Geometry: final body of the model. Coordinates: model frame, mm. A direction names the side the tool comes from. Give positions to 0.01 mm unless a question says otherwise; leave off trailing zeros. Write each loop counter-clockwise with the first axis right and the second up, starting at its lowest first coordinate (ties: lowest second). Pieces come first, ordered by that corner, then holes.
Q1. Cut plane D-D on y = 79. Return the cut outline in (x, z).
Q2. Cut plane A-A on z = -107.95. Return the cut outline in (x, y), plus the area to 3 significant figures.
Q3. Draft query along Z for faces 1 (the face through (-117.96, -25.13, -26.78)), 2 (the face through (107.683, -49.491, 63.856)), 3 (the face through (-114.478, -49.491, -70.117)), 4 (the face through (-120, -91.44, -112)). Return one class per face: pulls with the +Z half, pulls with the -Z half, needs draft (parallel to the pull), parting line crosses it, or undercut.
Q4. Pin query (flat end, axial travel): pin 1 (4 mm diameter, centred on x = -62, z = 95, fed in from +Y); pin 2 (3 mm diameter, centred on y = -2, z = 18.5, fed in from -X); pin 3 (14.5 mm diameter, centred on x = 107.95, z = 107.95, fed in from +Y); pin 4 (10 mm diameter, centred on x = 98.5, z = -73.5, fed in from -Y). Return the tip coordinate at first contact, or that it passes through.
Q5. Cut plane B-B on x = 0. Return the cut outline in (y, z).
Q6. Reachability of faces 5 (the face through (114, -6.35, -7)), 6 (the face through (-1, -104.14, 82)), 7 (the face through (-108, -91.44, 117)) from +Z, -Z, +X, -X, +Y, -Y: full face, straight path, thin tool, end or side. Return the list, or none.
Q7. Cut plane C-C on z = 107.95. Return the cut outline in (x, y), plus the area to 3 significant figures.
Q8. Line query: L1, parallel to X at y = -15.5, z = -40.5; L2, parallel to Z at x = 111.76, y = -35; L3, parallel to Y at x = 39.5, z = -5.5. Output: solid intervals per line, ascending.
```python
from build123d import *

# Parameters (mm, degrees)
SKETCH1_R                = 101.6
SKETCH1_R_2              = 88.9
BOSS_EXTRUDE1_DEPTH      = 38.1
SKETCH2_W                = 254
SKETCH2_H                = 177.8
BOSS_EXTRUDE2_DEPTH      = 12.7
BOSS_EXTRUDE3_REACH      = 275.106
BOSS_EXTRUDE3_END_RADIUS = 101.6
SKETCH3_W                = 203.2
SKETCH3_H                = 38.1
SKETCH10_W               = 25.4
SKETCH10_H               = 88.9
BOSS_EXTRUDE5_DEPTH      = 97.79
SKETCH11_R               = 6.35
CUT_EXTRUDE1_DEPTH       = 38.1
RIB3_START               = -38.1
RIB3_DEPTH               = 38.1
BOSS_EXTRUDE6_DEPTH      = 25.4
BOSS_EXTRUDE7_DEPTH      = 25.4
SKETCH17_R               = 6.35
CUT_EXTRUDE2_DEPTH       = 25.4


# Read off the part's stored shape, not the designer's step: Rib3
with BuildPart() as part:
    # Sketch1 → Boss-Extrude1 (new body)
    with BuildSketch(Plane.XY):
        with Locations(Location((0, 0, 0), (0, 0, 180))):
            Circle(SKETCH1_R)
        with Locations(Location((0, 0, 0), (0, 0, 180))):
            Circle(SKETCH1_R_2, mode=Mode.SUBTRACT)
    extrude(amount=BOSS_EXTRUDE1_DEPTH)



with BuildPart() as body_2:
    # Sketch2 → Boss-Extrude2 (new body)
    with BuildSketch(Plane(origin=(0, -116.84, 0), x_dir=(1, 0, 0), z_dir=(0, 1, 0))):
        with Locations((0, -38.1)):
            Rectangle(SKETCH2_W, SKETCH2_H)
    extrude(amount=BOSS_EXTRUDE2_DEPTH)


with BuildPart() as part_1:
    add(part.part)

    add(body_2.part)  # Boss-Extrude3 merges body 2
    # Boss-Extrude3: up to this cylinder (the profile starts outside it)
    boss_extrude3_end = Plane(origin=(0, 0, 19.05), z_dir=(0, 0, -1)) * Cylinder(BOSS_EXTRUDE3_END_RADIUS, 754.412, mode=Mode.PRIVATE)
    # Sketch3 → Boss-Extrude3 (add, up to the surface)
    with BuildSketch(Plane(origin=(0, -104.14, 0), x_dir=(1, 0, 0), z_dir=(0, 1, 0)), mode=Mode.PRIVATE) as boss_extrude3_sk1:
        with Locations((0, -19.05)):
            Rectangle(SKETCH3_W, SKETCH3_H)
    boss_extrude3_tool1 = extrude(boss_extrude3_sk1.sketch, amount=BOSS_EXTRUDE3_REACH, mode=Mode.PRIVATE) - boss_extrude3_end
    add(boss_extrude3_tool1.solids().sort_by_distance((0, -104.14, 19.05))[0])

    # Sketch10 → Boss-Extrude5 (add)
    with BuildSketch(Plane(origin=(0, -104.14, 0), x_dir=(1, 0, 0), z_dir=(0, 1, 0))):
        with Locations((-114.3, 6.35)):
            Rectangle(SKETCH10_W, SKETCH10_H)
    boss_extrude5 = extrude(amount=BOSS_EXTRUDE5_DEPTH)

    # Mirror1: Boss-Extrude5 across plane
    add(boss_extrude5.mirror(Plane(origin=(0, 0, 0), x_dir=(0, 0, 1), z_dir=(1, 0, 0))))

    # Sketch11 → Cut-Extrude1 (cut)
    with BuildSketch(Plane(origin=(0, -6.35, 0), x_dir=(1, 0, 0), z_dir=(0, 1, 0))):
        with Locations(Location((-111.76, 25.4, 0), (0, 0, 270))):
            Circle(SKETCH11_R)
    cut_extrude1 = extrude(amount=-CUT_EXTRUDE1_DEPTH, mode=Mode.SUBTRACT)

    # Mirror2: Cut-Extrude1 across plane
    add(cut_extrude1.mirror(Plane(origin=(0, 0, 0), x_dir=(0, 0, 1), z_dir=(1, 0, 0))), mode=Mode.SUBTRACT)

    # Rib3 outline → Rib3 (add)
    with BuildSketch(Plane.ZY.offset(127).offset(RIB3_START)):
        Polygon((127, -104.14), (127, -91.44), (88.9, -91.44), (38.1, -6.35), (38.1, -104.14), align=None)
    rib3 = extrude(amount=RIB3_DEPTH)

    # Mirror3: Rib3 across plane
    add(rib3.mirror(Plane(origin=(0, 0, 0), x_dir=(0, 0, 1), z_dir=(1, 0, 0))))

    # Sketch15 → Boss-Extrude6 (add)
    with BuildSketch(Plane.ZY.offset(127)):
        Polygon((-50.8, -6.35), (-50.8, -116.84), (-127, -116.84), (-127, -91.44), (-88.9, -91.44), align=None)
    extrude(amount=-BOSS_EXTRUDE6_DEPTH)

    # Sketch16 → Boss-Extrude7 (add)
    with BuildSketch(Plane(origin=(127, 0, 0), x_dir=(0, 0, -1), z_dir=(1, 0, 0))):
        Polygon((50.8, -6.35), (88.9, -91.44), (127, -91.44), (127, -116.84), (50.8, -116.84), align=None)
    extrude(amount=-BOSS_EXTRUDE7_DEPTH)

    # Sketch17 → Cut-Extrude2 (cut)
    with BuildSketch(Plane(origin=(0, -91.44, 0), x_dir=(1, 0, 0), z_dir=(0, 1, 0))):
        with Locations(Location((114.3, 107.95, 0), (0, 0, 270))):
            Circle(SKETCH17_R)
        with Locations(Location((-114.3, 107.95, 0), (0, 0, 270))):
            Circle(SKETCH17_R)
        with Locations(Location((-107.95, -107.95, 0), (0, 0, 270))):
            Circle(SKETCH17_R)
        with Locations(Location((107.95, -107.95, 0), (0, 0, 270))):
            Circle(SKETCH17_R)
    extrude(amount=-CUT_EXTRUDE2_DEPTH, mode=Mode.SUBTRACT)


solid = part_1.part
```
Data:
1. outline: (-63.89, 0) - (-40.77, 0) - (-40.77, 38.1) - (-63.89, 38.1) - close; (40.77, 0) - (63.89, 0) - (63.89, 38.1) - (40.77, 38.1) - close
2. outline: (-127, -116.84) - (-120.65, -116.84) - (-120.65, -91.44) - (-127, -91.44) - close; (-107.95, -116.84) - (-101.6, -116.84) - (-101.6, -91.44) - (-107.95, -91.44) - close; (101.6, -116.84) - (107.95, -116.84) - (107.95, -91.44) - (101.6, -91.44) - close; (120.65, -116.84) - (127, -116.84) - (127, -91.44) - (120.65, -91.44) - close
2. area: 645 mm2
3. face 1: undercut
3. face 2: pulls with the +Z half
3. face 3: pulls with the -Z half
3. face 4: needs draft
4. pin 1: stops at y = -104.14
4. pin 2: stops at x = -101.6
4. pin 3: stops at y = -91.44
4. pin 4: stops at y = -116.84
5. outline: (-116.84, -50.8) - (-104.14, -50.8) - (-104.14, 0) - (-88.9, 0) - (-88.9, 38.1) - (-104.14, 38.1) - (-104.14, 127) - (-116.84, 127) - close; (88.9, 0) - (101.6, 0) - (101.6, 38.1) - (88.9, 38.1) - close
6. face 5: +Z, -Z, +X, +Y
6. face 6: +Z, +Y
6. face 7: +Z, +X, -X, +Y
7. outline: (-127, -116.84) - (-114.3, -116.84) - (-114.3, -91.44) - (-127, -91.44) - close; (-101.6, -116.84) - (101.6, -116.84) - (101.6, -91.44) - (88.9, -91.44) - (88.9, -104.14) - (-88.9, -104.14) - (-88.9, -91.44) - (-101.6, -91.44) - close; (114.3, -116.84) - (127, -116.84) - (127, -91.44) - (114.3, -91.44) - close
7. area: 3,550 mm2
8. L1: x = -127 to -101.6, 101.6 to 127
8. L2: z = -63.63 to -31.75, -19.05 to 55.2
8. L3: y = -116.84 to -104.14
